```python
from build123d import *

# Parameters (mm, degrees)
F1_DEPTH = 177.8
F3_DEPTH = 3.175
F5_DEPTH = 3.175


with BuildPart() as f1:
    # F0 (on Front) → F1 (new body)
    with BuildSketch(Plane.XZ):
        with BuildLine():
            ThreePointArc((0, 9.525), (2.789808, 2.789808), (9.525, 0))
            Line((9.525, 0), (73.025, 0))
            ThreePointArc((73.025, 0), (79.760192, 2.789808), (82.55, 9.525))
            ThreePointArc((82.55, 9.525), (79.760192, 16.260192), (73.025, 19.05))
            Line((73.025, 19.05), (65.405, 19.05))
            Line((65.405, 19.05), (65.405, 15.875))
            Line((65.405, 15.875), (73.025, 15.875))
            ThreePointArc((73.025, 15.875), (77.515128, 14.015128), (79.375, 9.525))
            ThreePointArc((79.375, 9.525), (77.515128, 5.034872), (73.025, 3.175))
            Line((73.025, 3.175), (9.525, 3.175))
            ThreePointArc((9.525, 3.175), (5.034872, 5.034872), (3.175, 9.525))
            ThreePointArc((3.175, 9.525), (5.034872, 14.015128), (9.525, 15.875))
            Line((9.525, 15.875), (17.145, 15.875))
            Line((17.145, 15.875), (17.145, 19.05))
            Line((17.145, 19.05), (9.525, 19.05))
            ThreePointArc((9.525, 19.05), (2.789808, 16.260192), (0, 9.525))
        make_face()
    extrude(amount=F1_DEPTH)

    # F2 (on face) → F3 (join)
    with BuildSketch(Plane.XZ.offset(177.8)):
        with BuildLine():
            Line((73.025, 19.05), (9.525, 19.05))
            ThreePointArc((9.525, 19.05), (2.789808, 16.260192), (0, 9.525))
            ThreePointArc((0, 9.525), (2.789808, 2.789808), (9.525, 0))
            Line((9.525, 0), (73.025, 0))
            ThreePointArc((73.025, 0), (79.760192, 2.789808), (82.55, 9.525))
            ThreePointArc((82.55, 9.525), (79.760192, 16.260192), (73.025, 19.05))
        make_face()
    extrude(amount=F3_DEPTH)

    # F4 (on face) → F5 (join)
    with BuildSketch(Plane(origin=(0, 0, 0), x_dir=(-1, 0, 0), z_dir=(0, 1, 0))):
        with BuildLine():
            Line((-65.405, 9.525), (-65.405, 19.05))
            Line((-65.405, 19.05), (-73.025, 19.05))
            ThreePointArc((-73.025, 19.05), (-79.760192, 16.260192), (-82.55, 9.525))
            ThreePointArc((-82.55, 9.525), (-79.760192, 2.789808), (-73.025, 0))
            Line((-73.025, 0), (-9.525, 0))
            ThreePointArc((-9.525, 0), (-2.789808, 2.789808), (0, 9.525))
            ThreePointArc((0, 9.525), (-2.789808, 16.260192), (-9.525, 19.05))
            Line((-9.525, 19.05), (-17.145, 19.05))
            Line((-17.145, 19.05), (-17.145, 9.525))
            Line((-17.145, 9.525), (-65.405, 9.525))
        make_face()
    extrude(amount=F5_DEPTH)


solid = f1.part
```
The listing builds one solid part. Answer for the finished solid, in the listing's coordinates (mm). A direction names the side the tool comes from. Round coordinates to 2 decimals unless told otherwise and drop trailing zeros. Write each loop counter-clockwise with the first axis right and the second up, starting at its lowest first coordinate (ties: lowest second). Pieces come first, ordered by that corner, then holes. Notation, with made-up numbers: (57.25, -6) -> (100.25, -6) arc R26 ccw to (100.25, 32) -> close; hole circle Ø9 at (4.25, 47.25). An arc over 180 degrees is marked (long way). Answer as a JSON object with one key per item and string values. Group by question number.
Q1. Each of these flat-tipped pins is pushed along its axis until it touches: pin 1 Ø5 at (y, z) = (-108, 13.5) entering from -X; pin 2 Ø19 at (x, y) = (32, -112) entering from +Z (3 decimals); pin 3 Ø1.5 at (y, z) = (-74.5, 3.5) entering from +X. Where does it stop, or does it pass through?
Q2. Determine the mould class of faces 4 (the face through (41, -177.8, 11)), 5 (the face through (69, -88, 15.875)), 6 (the face through (41, -180.975, 10)) for opening direction X: pulls with the +X half, pulls with the -X half, needs draft (parallel to the pull), parting line crosses it, or undercut.
Q3. Which of the six approach directions +Z, -Z, +X, -X, +Y, -Y give full straight-line access (tool end or side, diameter ignored) to faces 1 (the face through (42, -90, 0)), 2 (the face through (42, -88, 3.175)), 3 (the face through (65.405, -88, 17))?
Q4. Section A-A (y = -29) is taken. Write down the section's boundary in (x, z) (3 decimals), plus the area to 3 significant figures.
Q5. Section B-B (x = 27) is taken. Write down the section's boundary in (y, z) (3 decimals).
Q6. Section C-C (z = 14) is taken. Write down the section's boundary in (x, y) (3 decimals).
Q7. Straight lines are drawn through the part: line 1 along Y through (x, z) = (67.5, 11) (3 decimals); line 2 along Z through (x, y) = (12, -16.5) (3 decimals); line 3 along X through (y, z) = (-106.5, 10). For each, find the intervals that lie inside material, in ascending order.
Check values:
{
 "1": {"pin 1": "x = 0.11", "pin 2": "z = 3.175", "pin 3": "x = 80.96"},
 "2": {"face 4": "undercut", "face 5": "undercut", "face 6": "needs draft"},
 "3": {"face 1": "-Z, +X, -X, +Y, -Y", "face 2": "none", "face 3": "+Z, +Y"},
 "4": {"outline": "(9.525, 0) -> (73.025, 0) arc R9.525 ccw to (73.025, 19.05) -> (65.405, 19.05) -> (65.405, 15.875) -> (73.025, 15.875) arc R6.35 cw to (73.025, 3.175) -> (9.525, 3.175) arc R6.35 cw to (9.525, 15.875) -> (17.145, 15.875) -> (17.145, 19.05) -> (9.525, 19.05) arc R9.525 ccw to start", "area": "408 mm^2"},
 "5": {"outline": "(-180.975, 0) -> (3.175, 0) -> (3.175, 9.525) -> (0, 9.525) -> (0, 3.175) -> (-177.8, 3.175) -> (-177.8, 19.05) -> (-180.975, 19.05) -> close"},
 "6": {"outline": "(1.117, -180.975) -> (81.433, -180.975) -> (81.433, 3.175) -> (65.405, 3.175) -> (65.405, 0) -> (77.53, 0) -> (77.53, -177.8) -> (5.02, -177.8) -> (5.02, 0) -> (17.145, 0) -> (17.145, 3.175) -> (1.117, 3.175) -> close"},
 "7": {"line 1": "-180.975 to -177.8, 0 to 3.175", "line 2": "0 to 3.175, 15.875 to 19.05", "line 3": "0.01 to 3.19, 79.36 to 82.54"}
}
